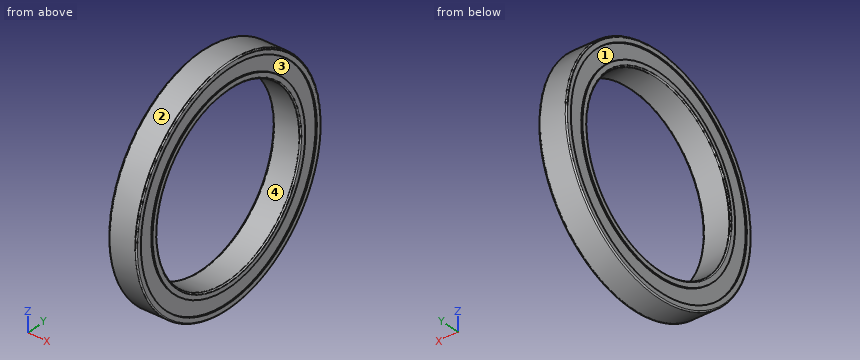
from build123d import *

# Parameters (mm, degrees)
FILLET1_R = 0.3
FILLET2_R = 0.3


with BuildPart() as part:
    # Sketch1 → Revolve1 (revolve)
    with BuildSketch(Plane.XY, mode=Mode.PRIVATE) as revolve1_sk:
        Polygon((0, 22.5), (7, 22.5), (7, 23.95), (6.68, 23.95), (6.68, 27.6), (7, 27.6), (7, 29), (0, 29), (0, 27.6), (0.32, 27.6), (0.32, 23.95), (0, 23.95), align=None)
    revolve(revolve1_sk.sketch.rotate(Axis((0, 0, 0), (1, 0, 0)), 90), axis=Axis((0, 0, 0), (1, 0, 0)))

    # Fillet1
    fillet1_edges = [part.edges().sort_by_distance(p)[0] for p in [
        (0, 0, -29),
        (7, 0, -29),
    ]]
    fillet(fillet1_edges, radius=FILLET1_R)

    # Fillet2
    fillet2_edges = [part.edges().sort_by_distance(p)[0] for p in [
        (7, 0, -22.5),
        (0, 0, -22.5),
    ]]
    fillet(fillet2_edges, radius=FILLET2_R)


solid = part.part
Could you check a few things on this model? Use its own coordinates, in mm. Face numbers are marked on the shaded views. A direction names the side the tool comes from. Coordinates: 2 decimals unless noted, no trailing zeros. Order: outer loops, then holes, each group sorted by start corner. A loop starts at its lowest first (then second) coordinate and runs counter-clockwise, first axis right, second up. Notation, with made-up numbers: (-3, 50.5) - (23, 50.5) arc R26 cw to (23, 72.5) - close; hole circle Ø5 at (78.5, 41). An arc over 180 degrees is marked (long way). Answer in a Markdown table with one row per item. Add a question column.
(1) Will these pins go through, and if not, where does the flat tip stop? pin 1 (1.5 mm diameter, centred on x = 6, y = 16, fed in from +Z); pin 2 (3 mm diameter, centred on x = 3.5, z = -4.5, fed in from -Y); pin 3 (3 mm diameter, centred on x = 5, z = 10, fed in from +Y).
(2) If we mould it in two halves opening along Z, with no side actions, what happens to the marked faces 1 and 2? For each: released by +Z, released by -Z, zero draft, split by the parting line, or undercut.
(3) I need wall thicknesses on L1, parallel to Y at x = 6.9, z = 0; L2, parallel to Y at x = 3, z = 0.5; L3, parallel to Y at x = 0.15, z = 0. Which ranges of each line are inside material? Lowest first, please.
(4) If we section it at C-C, the plane x = 2: Please give me the cut outline in (y, z), then the cut area to 3 significant figures.
(5) On a 3-axis mill with a long thin cutter (end or side, diameter ignored), from which of +Z, -Z, +X, -X, +Y, -Y can I reach the whole of each face in a straight line? I mean the marked faces 3 and 4. Say none if no direction works.
Results are:
| question | item | result |
|---|---|---|
| 1 | pin 1 | stops at z = 24.67 |
| 1 | pin 2 | stops at y = -28.84 |
| 1 | pin 3 | stops at y = 27.73 |
| 2 | face 1 | undercut |
| 2 | face 2 | split by the parting line |
| 3 | L1 | y = -28.92 to -27.6, -23.95 to -22.58, 22.58 to 23.95, 27.6 to 28.92 |
| 3 | L2 | y = -29 to -22.49, 22.49 to 29 |
| 3 | L3 | y = -28.96 to -27.6, -23.95 to -22.54, 22.54 to 23.95, 27.6 to 28.96 |
| 4 | outline | circle Ø58 at (0, 0); hole circle Ø45 at (0, 0) |
| 4 | area | 1,050 mm2 |
| 5 | face 3 | +X |
| 5 | face 4 | +X, -X |
